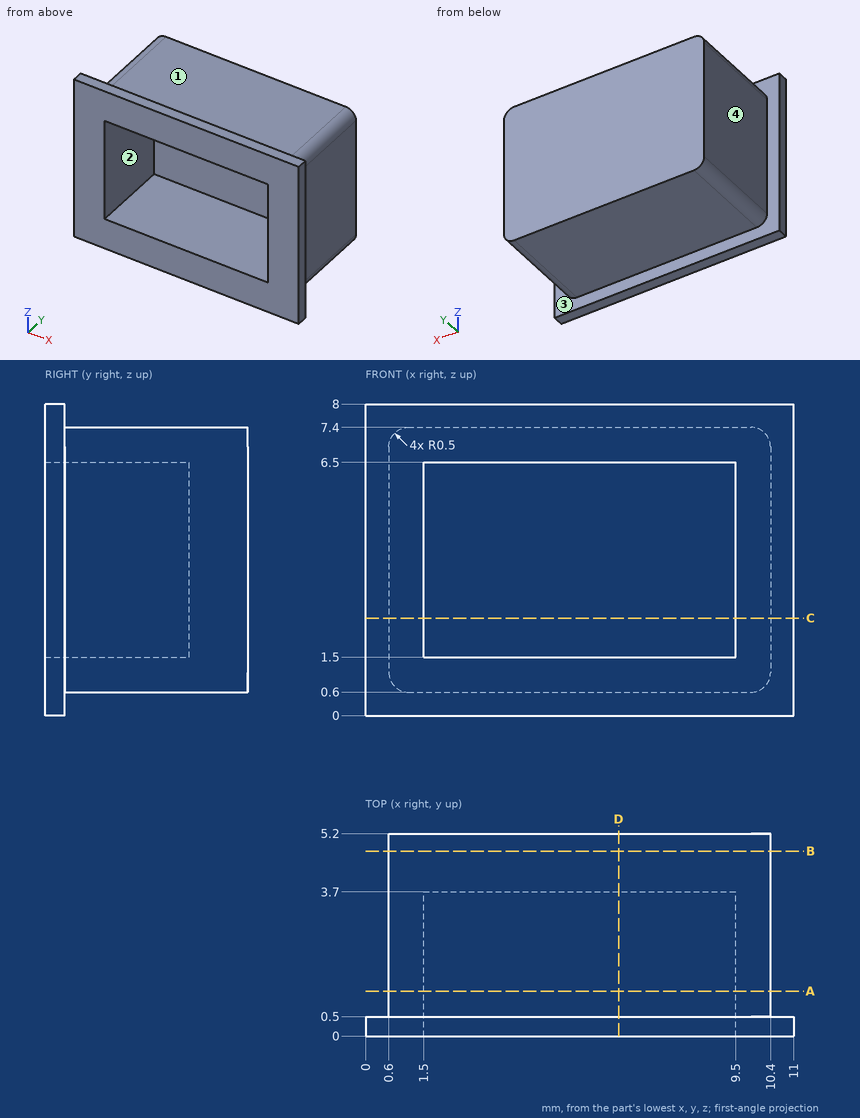
The drawing under review shows one solid part. Ordinate dimensions are in mm from its lowest x, y, z. A direction names the side the tool comes from. Coordinates: 2 decimals unless noted, no trailing zeros. Write each loop counter-clockwise with the first axis right and the second up, starting at its lowest first coordinate (ties: lowest second). Pieces come first, ordered by that corner, then holes.
1) Add section A-A (y = 1.15). Write out the cut boundary in (x, z).
2) Machinability: for the marked faces 1, 2, 3 and 4, which of the approach directions +Z, -Z, +X, -X, +Y, -Y give a long, thin tool a straight path to every point of the face, cutting with its end or side? Answer none if there is none.
3) To check wall thickness, follow L1, parallel to Z at x = 8.5, y = 0.55; L2, parallel to X at y = 0.9, z = 3.5; L3, parallel to Y at x = 5, z = 3.5. State the ranges of each line that lie inside material, in increasing order.
4) Insertion check: pin 1 (3 mm diameter, centred on x = 5, y = 4.5, fed in from -Z); pin 2 (2.5 mm diameter, centred on x = 7.5, y = 3.5, fed in from +Z); pin 3 (1.8 mm diameter, centred on y = 2, z = 4.5, fed in from -X). Each pin has a flat end and moves straight along its axis. Give the tip position at first contact, or say it passes through.
5) Add section D-D (x = 6.5). Write out the cut boundary in (y, z), plus the area to 3 significant figures.
6) Add section C-C (z = 2.5). Write out the cut boundary in (x, y).
7) Add section B-B (y = 4.75). Write out the cut boundary in (x, z).
Check result:
1. outline: (0.6, 1.1) arc R0.5 ccw to (1.1, 0.6) - (9.9, 0.6) arc R0.5 ccw to (10.4, 1.1) - (10.4, 6.9) arc R0.5 ccw to (9.9, 7.4) - (1.1, 7.4) arc R0.5 ccw to (0.6, 6.9) - close; hole (1.5, 1.5) - (9.5, 1.5) - (9.5, 6.5) - (1.5, 6.5) - close
2. face 1: +Z, +X, -X, +Y
2. face 2: -Y
2. face 3: +Y
2. face 4: +Z, -Z, -X, +Y
3. L1: z = 0.6 to 1.5, 6.5 to 7.4
3. L2: x = 0.6 to 1.5, 9.5 to 10.4
3. L3: y = 3.7 to 5.2
4. pin 1: stops at z = 0.6
4. pin 2: stops at z = 7.4
4. pin 3: stops at x = 0.6
5. outline: (0, 0) - (0.5, 0) - (0.5, 0.6) - (5.2, 0.6) - (5.2, 7.4) - (0.5, 7.4) - (0.5, 8) - (0, 8) - (0, 6.5) - (3.7, 6.5) - (3.7, 1.5) - (0, 1.5) - close
5. area: 17.5 mm2
6. outline: (0, 0) - (1.5, 0) - (1.5, 3.7) - (9.5, 3.7) - (9.5, 0) - (11, 0) - (11, 0.5) - (10.4, 0.5) - (10.4, 5.2) - (0.6, 5.2) - (0.6, 0.5) - (0, 0.5) - close
7. outline: (0.6, 1.1) arc R0.5 ccw to (1.1, 0.6) - (9.9, 0.6) arc R0.5 ccw to (10.4, 1.1) - (10.4, 6.9) arc R0.5 ccw to (9.9, 7.4) - (1.1, 7.4) arc R0.5 ccw to (0.6, 6.9) - close
